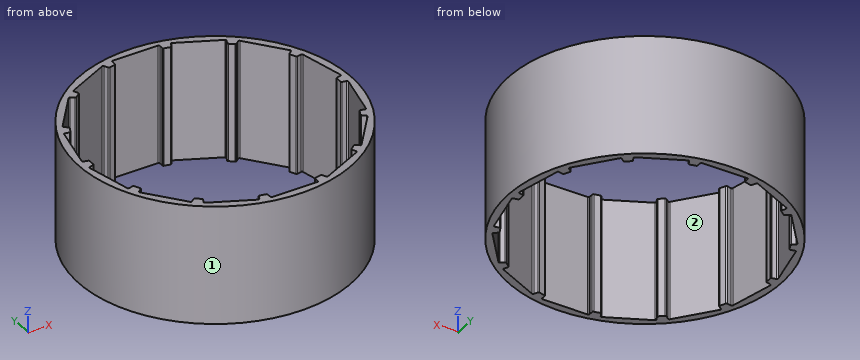
```python
from build123d import *

# Parameters (mm, degrees)
SKETCH_5_R               = 34.5
SKETCH_5_R_2             = 31.5
EXTRUDE_3_DEPTH          = 30
SKETCH_6_W               = 12.1
SKETCH_6_H               = 2
CUT_EXTRUDE_1_DEPTH      = 31
PATTERN_CIRCULAR_4_COUNT = 14
FILLET_1_R               = 0.3
FILLET_2_R               = 0.3
FILLET_3_R               = 0.3


with BuildPart() as part:
    # ｽｹｯﾁ5 → ﾎﾞｽ - 押し出し3 (new body)
    with BuildSketch(Plane.XY):
        Circle(SKETCH_5_R)
        Circle(SKETCH_5_R_2, mode=Mode.SUBTRACT)
    extrude(amount=EXTRUDE_3_DEPTH)

    # ｽｹｯﾁ6 → ｶｯﾄ - 押し出し1 (cut, through all)
    with BuildSketch(Plane.XY.offset(30)):
        with Locations((0, 31.5)):
            Rectangle(SKETCH_6_W, SKETCH_6_H)
    cut_extrude_1 = extrude(amount=-CUT_EXTRUDE_1_DEPTH, mode=Mode.SUBTRACT)

    # 円形ﾊﾟﾀｰﾝ4: ｶｯﾄ - 押し出し1 ×14 about axis
    pattern_circular_4_axis = Axis((0, 0, 0), (0, 0, 1))
    for i in range(1, PATTERN_CIRCULAR_4_COUNT):
        add(cut_extrude_1.rotate(pattern_circular_4_axis, i * 360 / PATTERN_CIRCULAR_4_COUNT), mode=Mode.SUBTRACT)

    # ﾌｨﾚｯﾄ1
    fillet_1_edges = [part.edges().sort_by_distance(p)[0] for p in [
        (-6.05, 30.91354881, 15),
        (-6.05, 32.5, 15),
        (-8.650359871, 31.906484828, 15),
        (-7.962024496, 30.477141695, 15),
    ]]
    fillet(fillet_1_edges, radius=FILLET_1_R)

    # ﾌｨﾚｯﾄ2
    fillet_2_edges = [part.edges().sort_by_distance(p)[0] for p in [
        (6.05, 30.91354881, 15),
        (19.552083172, -26.656491585, 15),
        (21.637409879, -24.993499029, 15),
        (29.181636481, -15.533338091, 15),
        (6.05, 32.5, 15),
        (30.338905495, -13.130244222, 15),
        (33.031408796, -1.333616485, 15),
        (33.031408796, 1.333616485, 15),
        (30.338905495, 13.130244222, 15),
        (29.181636481, 15.533338091, 15),
        (21.637409879, 24.993499029, 15),
        (19.552083172, 26.656491585, 15),
        (8.650359871, 31.906484828, 15),
        (7.962024496, 30.477141695, 15),
        (18.863747798, 25.227148452, 15),
        (20.397072393, 24.004362891, 15),
        (27.941298995, 14.544201953, 15),
        (28.792229949, 12.777225622, 15),
        (31.484733249, 0.980597884, 15),
        (31.484733249, -0.980597884, 15),
        (28.792229949, -12.777225622, 15),
        (27.941298995, -14.544201953, 15),
        (20.397072393, -24.004362891, 15),
        (18.863747798, -25.227148452, 15),
    ]]
    fillet(fillet_2_edges, radius=FILLET_2_R)

    # ﾌｨﾚｯﾄ3
    fillet_3_edges = [part.edges().sort_by_distance(p)[0] for p in [
        (-30.338905495, 13.130244222, 15),
        (-33.031408796, 1.333616485, 15),
        (-33.031408796, -1.333616485, 15),
        (-30.338905495, -13.130244222, 15),
        (-29.181636481, -15.533338091, 15),
        (-21.637409879, -24.993499029, 15),
        (-19.552083172, -26.656491585, 15),
        (-8.650359871, -31.906484828, 15),
        (-6.05, -32.5, 15),
        (6.05, -32.5, 15),
        (8.650359871, -31.906484828, 15),
        (-19.552083172, 26.656491585, 15),
        (-18.863747798, 25.227148452, 15),
        (7.962024496, -30.477141695, 15),
        (6.05, -30.91354881, 15),
        (-6.05, -30.91354881, 15),
        (-7.962024496, -30.477141695, 15),
        (-18.863747798, -25.227148452, 15),
        (-20.397072393, -24.004362891, 15),
        (-27.941298995, -14.544201953, 15),
        (-28.792229949, -12.777225622, 15),
        (-31.484733249, -0.980597884, 15),
        (-31.484733249, 0.980597884, 15),
        (-28.792229949, 12.777225622, 15),
        (-27.941298995, 14.544201953, 15),
        (-20.397072393, 24.004362891, 15),
        (-21.637409879, 24.993499029, 15),
        (-29.181636481, 15.533338091, 15),
    ]]
    fillet(fillet_3_edges, radius=FILLET_3_R)


solid = part.part
```
Verification items for the finished model (mm, model axes). Face numbers are marked on the shaded views. Coordinates: 2 decimals unless noted, no trailing zeros. Loops run counter-clockwise (first coordinate to the right, second up) from the corner with the lowest first, then second, coordinate; pieces in that order, holes last. Notation, with made-up numbers: (27.25, 15) -> (32.25, 15) arc R8 ccw to (32.25, 29) -> close; hole circle Ø2 at (22, 36). An arc over 180 degrees is marked (long way). Answer in a Markdown table with one row per item. Add a question column.
1. Draft check along X on the marked faces 1 and 2. Enter one of: +X half, -X half, draft (parallel to the pull), parting line (faces both ways), or undercut.
2. Depth check by flat-ended pin: P1, Ø3, axis at x = 27.5, z = 9, coming from the +Y side; P2, Ø12, axis at x = -27.5, z = 16.5, coming from the +Y side; P3, Ø4, axis at x = -16.5, z = 8, coming from the -Y side. Enter the tip coordinate at first touch or a pass-through.
3. Section check A-A, the plane x = 0. Enter the section's corners in (y, z), then the cut area to 3 significant figures.
4. Section check B-B, the plane y = 6.5. Enter the section's corners in (x, z), then the cut area to 3 significant figures.
5. Material ranges on probe 1 along Y at (x, z) = (29, 26); probe 2 along Y at (x, z) = (20, 13); probe 3 along Y at (x, z) = (26.5, 5), recorded low to high. Write a range as [from, to].
Derived:
| question | item | result |
|---|---|---|
| 1 | face 1 | parting line |
| 1 | face 2 | undercut |
| 2 | P1 | stops at y = 22.68 |
| 2 | P2 | stops at y = 26.98 |
| 2 | P3 | stops at y = -31.3 |
| 3 | outline | (-34.5, 0) -> (-32.5, 0) -> (-32.5, 30) -> (-34.5, 30) -> close; (32.5, 0) -> (34.5, 0) -> (34.5, 30) -> (32.5, 30) -> close |
| 3 | area | 120 mm² |
| 4 | outline | (-33.88, 0) -> (-31.85, 0) -> (-31.85, 30) -> (-33.88, 30) -> close; (31.85, 0) -> (33.88, 0) -> (33.88, 30) -> (31.85, 30) -> close |
| 4 | area | 122 mm² |
| 5 | probe 1 | y = [-18.69, -15.76], [-15.4, -12.83], [12.83, 15.4], [15.76, 18.69] |
| 5 | probe 2 | y = [-28.11, -24.34], [24.34, 28.11] |
| 5 | probe 3 | y = [-22.09, -18.9], [18.9, 22.09] |
